The listing builds one solid part. Answer for the finished solid, in the listing's coordinates (mm). Give positions to 0.01 mm unless a question says otherwise; leave off trailing zeros. Loops run counter-clockwise (first coordinate to the right, second up) from the corner with the lowest first, then second, coordinate; pieces in that order, holes last.
Item 1: Section C-C, the plane y = 2.85 is taken. Give the vertices of the cut face in (x, z).
Item 2: This flat-tipped pin is pushed along its axis until it touches: pin 1 Ø2.5 at (x, z) = (-5, -5) entering from +Y. Where does it stop, or does it pass through?
Item 3: Consider line 1 along Z through (x, y) = (-5, 1.45); line 2 along Z through (x, y) = (-5.5, 3.95). Determine where each line is inside the solid, lowest interval first.
Item 4: Section A-A, the plane x = -5 is taken. Give the vertices of the cut face in (y, z), and give its area (3 significant figures).
Item 5: The mould has two halves that part along X. Classify faces 1 (the face through (-6.386, 2.465, -10.425)), 2 (the face through (0, 2, -25)), 3 (the face through (-6.386, 2.465, -4.425)), 4 (the face through (-5, 0, -25)): pulls with the +X half, pulls with the -X half, needs draft (parallel to the pull), parting line crosses it, or undercut.
Item 6: Section B-B, the plane z = -5 is taken. Give the vertices of the cut face in (x, y).
Autodesk Inventor part; units mm, degrees
ref_plane "YZ Plane" through (0, 0, 0) normal (1, 0, 0) x (0, 1, 0)
ref_plane "XZ Plane" through (0, 0, 0) normal (0, 1, 0) x (-1, 0, 0)
ref_plane "XY Plane" through (0, 0, 0) normal (0, 0, 1) x (1, 0, 0)
sketch "Sketch1" plane through (0, 0, 0) normal (0, 1, 0) x (-1, 0, 0)
  line L0 (0, 0) -> (10, 0)
  line L1 (10, 0) -> (10, -50)
  line L2 (10, -50) -> (0, -50)
  line L3 (0, -50) -> (0, 0)
  circle A0 centre (5, -5) radius 1.5
  circle A1 centre (5, -11) radius 1.5
  dimension "d0" = 10
  dimension "d1" = 50
  dimension "d4" = 3
  dimension "d5" = 3
  dimension "d6" = 6
  dimension "d7" = 5
  dimension "d8" = 5
extrude "Extrusion2" add sketch "Sketch1" along normal blind 5
properties part number "Soporte3_Dos"
Worked answers:
1. outline: (-10, -50) - (0, -50) - (0, 0) - (-10, 0) - close; hole circle Ø3 at (-5, -11); hole circle Ø3 at (-5, -5)
2. pin 1: passes through
3. line 1: z = -50 to -12.5, -9.5 to -6.5, -3.5 to 0
3. line 2: z = -50 to -12.41, -9.59 to -6.41, -3.59 to 0
4. outline: (0, -50) - (5, -50) - (5, -12.5) - (0, -12.5) - close; (0, -9.5) - (5, -9.5) - (5, -6.5) - (0, -6.5) - close; (0, -3.5) - (5, -3.5) - (5, 0) - (0, 0) - close
4. area: 220 mm2
5. face 1: undercut
5. face 2: pulls with the +X half
5. face 3: undercut
5. face 4: needs draft
6. outline: (-10, 0) - (-6.5, 0) - (-6.5, 5) - (-10, 5) - close; (-3.5, 0) - (0, 0) - (0, 5) - (-3.5, 5) - close
